The model under review builds one solid part; all positions refer to its coordinate system, in mm. A direction names the side the tool comes from. Coordinates: 2 decimals unless noted, no trailing zeros. Order: outer loops, then holes, each group sorted by start corner. A loop starts at its lowest first (then second) coordinate and runs counter-clockwise, first axis right, second up. Notation, with made-up numbers: (55.25, -40) -> (114.25, -40) arc R20 cw to (114.25, -18) -> close; hole circle Ø11 at (84.25, 77). An arc over 180 degrees is marked (long way). Put each result on its own line as item: value.
from build123d import *

# Parameters (mm, degrees)
SKETCH_1_R          = 16.5
SKETCH_1_R_2        = 14.5
EXTRUDE_1_DEPTH     = 35
SKETCH_3_R          = 16.5
EXTRUDE_2_DEPTH     = 2
SKETCH_4_W          = 49.747728002
SKETCH_4_H          = 43.690708299
CUT_EXTRUDE_1_DEPTH = 49.40970977
CUT_EXTRUDE_2_REACH = 45.744
SKETCH_5_R          = 3.75
FILLET_1_R          = 6


with BuildPart() as part:
    # 草图1 → 凸台-拉伸1 (new body)
    with BuildSketch(Plane(origin=(0, 0, 0), x_dir=(1, 0, 0), z_dir=(0, 1, 0))):
        with Locations(Location((0, 0, 0), (0, 0, 270))):
            Circle(SKETCH_1_R)
        with Locations(Location((0, 0, 0), (0, 0, 270))):
            Circle(SKETCH_1_R_2, mode=Mode.SUBTRACT)
    extrude(amount=EXTRUDE_1_DEPTH)

    # 草图3 → 凸台-拉伸2 (add)
    with BuildSketch(Plane(origin=(0, 35, 0), x_dir=(1, 0, 0), z_dir=(0, 1, 0))):
        with Locations(Location((0, 0, 0), (0, 0, 270))):
            Circle(SKETCH_3_R)
    extrude(amount=EXTRUDE_2_DEPTH)

    # 草图4 → 切除-拉伸1 (cut, through all)
    with BuildSketch(Plane.XY.offset(10)):
        with Locations((3.540684312, 17.876483266)):
            Rectangle(SKETCH_4_W, SKETCH_4_H)
    extrude(amount=CUT_EXTRUDE_1_DEPTH, mode=Mode.SUBTRACT)

    # 草图5 → 切除-拉伸2 (cut, up to next)
    with BuildSketch(Plane(origin=(0, 37, 0), x_dir=(1, 0, 0), z_dir=(0, 1, 0)), mode=Mode.PRIVATE) as cut_extrude_2_sk1:
        with Locations(Location((0, 0, 0), (0, 0, 270))):
            Circle(SKETCH_5_R)
    cut_extrude_2_tool1 = extrude(cut_extrude_2_sk1.sketch, amount=-CUT_EXTRUDE_2_REACH, mode=Mode.PRIVATE) & part.part
    add(cut_extrude_2_tool1.solids().sort_by_distance((0, 37, 0))[0], mode=Mode.SUBTRACT)

    # 圆角1
    fillet_1_edges = [part.edges().sort_by_distance(p)[0] for p in [
        (13.124404748, 18.5, 10),
        (-13.124404748, 18.5, 10),
    ]]
    fillet(fillet_1_edges, radius=FILLET_1_R)


solid = part.part
Item 1: Consider section C-C on x = 12. Write out the cut boundary in (y, z), and give its area (3 significant figures).
Answers below:
outline: (0, -11.32) -> (37, -11.32) -> (37, 9.55) -> (0, 9.55) -> (0, 8.14) -> (35, 8.14) -> (35, -8.14) -> (0, -8.14) -> close
area: 202 mm^2
Item 2: For pin 1 Ø4 at (x, z) = (4.5, -2.5) entering from -Y; pin 2 Ø1.5 at (y, z) = (11.5, -3.5) entering from -X; pin 3 Ø5 at (x, y) = (13, 10) entering from -Z, all flat-tipped, find the tip position at first contact; note any pin that passes through.
Answers below:
pin 1: y = 35
pin 2: x = -16.27
pin 3: z = -12.73
Item 3: For faces 1 (the flat face through (3.4, 35, -2.4)), 2 (the cylindrical face through (0.453, 18.241, -16.494)), list the 3-axis set-ups (+Z, -Z, +X, -X, +Y, -Y) from which the entire face can be reached by the end or side of a thin tool; tool diameter is ignored.
Answers below:
face 1: -Y
face 2: +Y, -Y
Item 4: Consider section A-A on z = 0. Write out the cut boundary in (x, y).
Answers below:
outline: (-16.5, 0) -> (-14.5, 0) -> (-14.5, 35) -> (-3.75, 35) -> (-3.75, 37) -> (-16.5, 37) -> close; (3.75, 35) -> (14.5, 35) -> (14.5, 0) -> (16.5, 0) -> (16.5, 37) -> (3.75, 37) -> close
Item 5: For line 1 (X direction, y = 35.8, z = 0); line 2 (X direction, y = 10.5, z = 0); line 3 (Y direction, x = -11, z = 1.25), list the stretches that pass through material, from the lowest coordinate up. Write a range as from..to.
Answers below:
line 1: -16.5..-3.75, 3.75..16.5
line 2: -16.5..-14.5, 14.5..16.5
line 3: 35..37
Item 6: Consider section D-D on z = 3. Write out the cut boundary in (x, y), and give its area (3 significant figures).
Answers below:
outline: (-16.22, 0) -> (-14.19, 0) -> (-14.19, 35) -> (-2.25, 35) -> (-2.25, 37) -> (-16.22, 37) -> close; (2.25, 35) -> (14.19, 35) -> (14.19, 0) -> (16.22, 0) -> (16.22, 37) -> (2.25, 37) -> close
area: 199 mm^2
Item 7: Mouldability with a two-part tool opening along X and no side actions: class faces 3 (the cylindrical face through (0.472, 17.255, -14.492)), 4 (the flat face through (-3, 37, -3)), 5 (the cylindrical face through (-13.087, 18.241, 8.958)) as +X half, -X half, draft (parallel to the pull), parting line (faces both ways), or undercut.
Answers below:
face 3: undercut
face 4: draft
face 5: -X half
Item 8: Consider section B-B on x = 0. Write out the cut boundary in (y, z), and give its area (3 significant figures).
Answers below:
outline: (0, -16.5) -> (37, -16.5) -> (37, -3.75) -> (35, -3.75) -> (35, -14.5) -> (0, -14.5) -> close; (35, 3.75) -> (37, 3.75) -> (37, 10) -> (35, 10) -> close
area: 108 mm^2
